```python
from build123d import *

# Parameters (mm, degrees)
F0_W     = 89.31
F0_H     = 48.5
F1_DEPTH = 18.8
F2_R     = 4.73
F3_DEPTH = 0.5
F4_R     = 5
F6_DEPTH = 14.78
F8_DEPTH = 14.78


with BuildPart() as f1:
    # F0 (on Top) → F1 (new body)
    with BuildSketch(Plane.XY):
        Rectangle(F0_W, F0_H)
    extrude(amount=F1_DEPTH)

    # F2 (on face) → F3 (join)
    with BuildSketch(Plane.XY.offset(18.8)):
        with Locations((-26.7, 11.9)):
            Circle(F2_R)
        with Locations((-26.7, -11.9)):
            Circle(F2_R)
        with Locations((-8.9, 11.9)):
            Circle(F2_R)
        with Locations((-8.9, -11.9)):
            Circle(F2_R)
        with Locations((8.9, 11.9)):
            Circle(F2_R)
        with Locations((8.9, -11.9)):
            Circle(F2_R)
        with Locations((26.7, 11.9)):
            Circle(F2_R)
        with Locations((26.7, -11.9)):
            Circle(F2_R)
    extrude(amount=F3_DEPTH)

    # F4
    f4_edges = [f1.edges().sort_by_distance(p)[0] for p in [
        (-44.655, 24.25, 9.4),
        (-44.655, -24.25, 9.4),
        (44.655, -24.25, 9.4),
        (44.655, 24.25, 9.4),
    ]]
    fillet(f4_edges, radius=F4_R)

    # F5 (on Top) → F6 (join)
    with BuildSketch(Plane.XY):
        with BuildLine():
            Line((45.75, 5.8), (44.655, 5.8))
            Line((44.655, 5.8), (44.655, -5.8))
            Line((44.655, -5.8), (45.75, -5.8))
            ThreePointArc((45.75, -5.8), (49.285534, -4.335534), (50.75, -0.8))
            Line((50.75, -0.8), (50.75, 0.8))
            ThreePointArc((50.75, 0.8), (49.285534, 4.335534), (45.75, 5.8))
        make_face()
    extrude(amount=F6_DEPTH)

    # F7 (on Top) → F8 (join)
    with BuildSketch(Plane.XY):
        with BuildLine():
            ThreePointArc((-50.75, 10.8), (-49.285534, 7.264466), (-45.75, 5.8))
            Line((-45.75, 5.8), (-44.655, 5.8))
            Line((-44.655, 5.8), (-44.655, 17.4))
            Line((-44.655, 17.4), (-45.75, 17.4))
            ThreePointArc((-45.75, 17.4), (-49.285534, 15.935534), (-50.75, 12.4))
            Line((-50.75, 12.4), (-50.75, 10.8))
        make_face()
        with BuildLine():
            Line((-45.75, -17.4), (-44.655, -17.4))
            Line((-44.655, -17.4), (-44.655, -5.8))
            Line((-44.655, -5.8), (-45.75, -5.8))
            ThreePointArc((-45.75, -5.8), (-49.285534, -7.264466), (-50.75, -10.8))
            Line((-50.75, -10.8), (-50.75, -12.4))
            ThreePointArc((-50.75, -12.4), (-49.285534, -15.935534), (-45.75, -17.4))
        make_face()
    extrude(amount=F8_DEPTH)


solid = f1.part
```
Read the model definition and answer for the solid it produces. Units are mm, in the model's axes. A direction names the side the tool comes from. Round coordinates to 2 decimals unless told otherwise and drop trailing zeros. Write each loop counter-clockwise with the first axis right and the second up, starting at its lowest first coordinate (ties: lowest second). Pieces come first, ordered by that corner, then holes. Notation, with made-up numbers: (23, 41.25) -> (60, 41.25) arc R27 ccw to (60, 68.25) -> close; hole circle Ø7 at (51, 54.5). An arc over 180 degrees is marked (long way). Answer in a Markdown table with one row per item. Add a question column.
1) Find section C-C, the plane z = 16.5. Determine the outline of the cut face in (x, y) (3 decimals).
2) Determine the mould class of faces 4 (the face through (49.25, -4.37, 7.29)), 5 (the face through (-1, 24.25, 9)), 6 (the face through (27, 12, 19.3)), 7 (the face through (-6.36, 15.89, 19.05)) for opening direction Y: pulls with the +Y half, pulls with the -Y half, needs draft (parallel to the pull), parting line crosses it, or undercut.
3) Find section B-B, the plane z = 2.5. Determine the outline of the cut face in (x, y) (3 decimals).
4) Consider line 1 (Z direction, x = 37, y = 21); line 2 (X direction, y = -16, z = 18) (3 decimals); line 3 (X direction, y = -22, z = 7.25). Determine where each line is inside the solid, lowest interval first.
5) Given P1, Ø1.8, axis at x = -47.5, y = -9, coming from the +Z side; P2, Ø3, axis at x = -2, y = 17.5, coming from the +Z side; P3, Ø0.5, axis at x = -45.5, z = 9.5, coming from the -Y side, each flat-ended and moving along its own axis, determine where each tip first touches the part or whether it passes through.
6) Find section A-A, the plane x = -26.7. Determine the outline of the cut face in (y, z), and give its area (3 significant figures).
7) Find section D-D, the plane x = 8.5. Determine the outline of the cut face in (y, z).
8) Which of the six approach directions +Z, -Z, +X, -X, +Y, -Y give full straight-line access (tool end or side, diameter ignored) to faces 1 (the face through (-47, -12, 14.78)), 2 (the face through (-1, 0, 18.8)), 3 (the face through (-43.229, -22.746, 9.532))?
Findings below:
| question | item | result |
|---|---|---|
| 1 | outline | (-44.655, -19.25) arc R5 ccw to (-39.655, -24.25) -> (39.655, -24.25) arc R5 ccw to (44.655, -19.25) -> (44.655, 19.25) arc R5 ccw to (39.655, 24.25) -> (-39.655, 24.25) arc R5 ccw to (-44.655, 19.25) -> close |
| 2 | face 4 | pulls with the -Y half |
| 2 | face 5 | pulls with the +Y half |
| 2 | face 6 | needs draft |
| 2 | face 7 | undercut |
| 3 | outline | (-50.75, -12.4) arc R5 ccw to (-45.75, -17.4) -> (-44.655, -17.4) -> (-44.655, -19.25) arc R5 ccw to (-39.655, -24.25) -> (39.655, -24.25) arc R5 ccw to (44.655, -19.25) -> (44.655, -5.8) -> (45.75, -5.8) arc R5 ccw to (50.75, -0.8) -> (50.75, 0.8) arc R5 ccw to (45.75, 5.8) -> (44.655, 5.8) -> (44.655, 19.25) arc R5 ccw to (39.655, 24.25) -> (-39.655, 24.25) arc R5 ccw to (-44.655, 19.25) -> (-44.655, 17.4) -> (-45.75, 17.4) arc R5 ccw to (-50.75, 12.4) -> (-50.75, 10.8) arc R5 ccw to (-45.75, 5.8) -> (-44.655, 5.8) -> (-44.655, -5.8) -> (-45.75, -5.8) arc R5 ccw to (-50.75, -10.8) -> close |
| 4 | line 1 | 0 to 18.8 |
| 4 | line 2 | -44.655 to 44.655 |
| 4 | line 3 | -43.83 to 43.83 |
| 5 | P1 | z = 14.78 |
| 5 | P2 | z = 18.8 |
| 5 | P3 | y = -17.4 |
| 6 | outline | (-24.25, 0) -> (24.25, 0) -> (24.25, 18.8) -> (16.63, 18.8) -> (16.63, 19.3) -> (7.17, 19.3) -> (7.17, 18.8) -> (-7.17, 18.8) -> (-7.17, 19.3) -> (-16.63, 19.3) -> (-16.63, 18.8) -> (-24.25, 18.8) -> close |
| 6 | area | 921 mm² |
| 7 | outline | (-24.25, 0) -> (24.25, 0) -> (24.25, 18.8) -> (16.61, 18.8) -> (16.61, 19.3) -> (7.19, 19.3) -> (7.19, 18.8) -> (-7.19, 18.8) -> (-7.19, 19.3) -> (-16.61, 19.3) -> (-16.61, 18.8) -> (-24.25, 18.8) -> close |
| 8 | face 1 | +Z, -X, +Y, -Y |
| 8 | face 2 | +Z |
| 8 | face 3 | +Z, -Z, -X, -Y |
